Read the model definition and answer for the solid it produces. Units are mm, in the model's axes. Give positions to 0.01 mm unless a question says otherwise; leave off trailing zeros. Write each loop counter-clockwise with the first axis right and the second up, starting at its lowest first coordinate (ties: lowest second). Pieces come first, ordered by that corner, then holes.
```python
from build123d import *

# Parameters (mm, degrees)
BOSS_EXTRUDE1_DEPTH = 6.35
SKETCH2_R           = 12.7
SKETCH2_R_2         = 5.159375
CUT_EXTRUDE1_DEPTH  = 59.887477446


with BuildPart() as part:
    # Sketch1 → Boss-Extrude1 (new body)
    with BuildSketch(Plane(origin=(0, 0, 0), x_dir=(1, 0, 0), z_dir=(0, 1, 0))):
        with BuildLine():
            Line((-25.4, 44.45), (25.4, 44.45))
            ThreePointArc((25.4, 44.45), (34.380256121, 40.730256121), (38.1, 31.75))
            Line((38.1, 31.75), (38.1, -31.75))
            ThreePointArc((38.1, -31.75), (34.380256121, -40.730256121), (25.4, -44.45))
            Line((25.4, -44.45), (-25.4, -44.45))
            ThreePointArc((-25.4, -44.45), (-34.380256121, -40.730256121), (-38.1, -31.75))
            Line((-38.1, -31.75), (-38.1, 31.75))
            ThreePointArc((-38.1, 31.75), (-34.380256121, 40.730256121), (-25.4, 44.45))
        make_face()
    extrude(amount=BOSS_EXTRUDE1_DEPTH)

    # Sketch2 → Cut-Extrude1 (cut, through all)
    with BuildSketch(Plane(origin=(0, 6.35, 0), x_dir=(1, 0, 0), z_dir=(0, 1, 0))):
        with Locations(Location((0, 19.05, 0), (0, 0, 270))):
            Circle(SKETCH2_R)
        with Locations(Location((-12.7, -31.75, 0), (0, 0, 270))):
            Circle(SKETCH2_R_2)
        with Locations(Location((12.7, -31.75, 0), (0, 0, 90))):
            Circle(SKETCH2_R_2)
    extrude(amount=-CUT_EXTRUDE1_DEPTH, mode=Mode.SUBTRACT)


solid = part.part
```
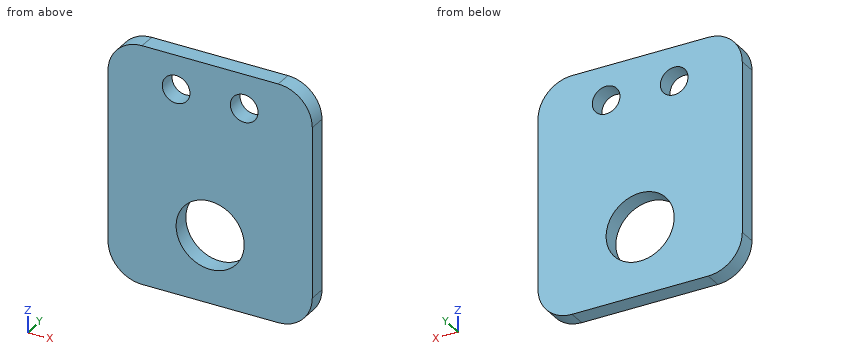
Item 1: Section D-D (z = 29.5) is taken. Write down the section's boundary in (x, y).
Result set:
outline: (-38.1, 0) - (-17.34, 0) - (-17.34, 6.35) - (-38.1, 6.35) - close; (-8.06, 0) - (8.06, 0) - (8.06, 6.35) - (-8.06, 6.35) - close; (17.34, 0) - (38.1, 0) - (38.1, 6.35) - (17.34, 6.35) - close
Item 2: Find the intervals of material crossed by line 1 along X through (y, z) = (4.25, 31.75); line 2 along X through (y, z) = (4.5, -19.05); line 3 along Z through (x, y) = (-16, 1.75), in increasing order.
Result set:
line 1: x = -38.1 to -17.86, -7.54 to 7.54, 17.86 to 38.1
line 2: x = -38.1 to -12.7, 12.7 to 38.1
line 3: z = -44.45 to 27.78, 35.72 to 44.45
Item 3: Section A-A (z = -19.05) is taken. Write down the section's boundary in (x, y), and give its area (3 significant figures).
Result set:
outline: (-38.1, 0) - (-12.7, 0) - (-12.7, 6.35) - (-38.1, 6.35) - close; (12.7, 0) - (38.1, 0) - (38.1, 6.35) - (12.7, 6.35) - close
area: 323 mm2
Item 4: Section B-B (x = 0) is taken. Write down the section's boundary in (y, z), and give its area (3 significant figures).
Result set:
outline: (0, -44.45) - (6.35, -44.45) - (6.35, -31.75) - (0, -31.75) - close; (0, -6.35) - (6.35, -6.35) - (6.35, 44.45) - (0, 44.45) - close
area: 403 mm2
Item 5: Section C-C (y = 2) is taken. Write down the section's boundary in (x, z).
Result set:
outline: (-38.1, -31.75) arc R12.7 ccw to (-25.4, -44.45) - (25.4, -44.45) arc R12.7 ccw to (38.1, -31.75) - (38.1, 31.75) arc R12.7 ccw to (25.4, 44.45) - (-25.4, 44.45) arc R12.7 ccw to (-38.1, 31.75) - close; hole circle Ø10.32 at (-12.7, 31.75); hole circle Ø25.4 at (0, -19.05); hole circle Ø10.32 at (12.7, 31.75)
